from build123d import *

# Parameters (mm, degrees)
BOSS_EXTRUDE1_DEPTH     = 40
SKETCH2_R               = 1.5
CUT_EXTRUDE1_DEPTH      = 40
SKETCH3_W               = 40
SKETCH3_H               = 54.5
SKETCH3_W_2             = 29
SKETCH3_H_2             = 46.5
BOSS_EXTRUDE2_DEPTH     = 18
SKETCH4_W               = 29
SKETCH4_H               = 46.5
CUT_EXTRUDE2_DEPTH      = 40
CUT_EXTRUDE3_DEPTH      = 137.090235877
CUT_EXTRUDE3_DEPTH_BACK = 137.090235877
SKETCH5_R               = 1.55
SKETCH5_R_2             = 1.05
FILLET1_R               = 20
FILLET2_R               = 20
FILLET3_R               = 20
CHAMFER1_SIZE           = 2


# Some blends are built 0.0001 mm under size
with BuildPart() as part:
    # Sketch1 → Boss-Extrude1 (new body)
    with BuildSketch(Plane.XY):
        Polygon((-63.639610307, 63.639610307), (0, 0), (0, 6), (2.485281374, 6), (-59.39696962, 67.882250994), align=None)
        Polygon((0, 6), (0, 0), (4.242640687, 4.242640687), (2.485281374, 6), align=None)
        Polygon((4.242640687, 4.242640687), (0, 0), (65, 0), (60.757359313, 4.242640687), (62.514718626, 6), (2.485281374, 6), align=None)
        Polygon((60.757359313, 4.242640687), (65, 0), (65, 6), (62.514718626, 6), align=None)
        Polygon((65, 6), (65, 0), (110.961940777, 45.961940777), (106.71930009, 50.204581464), (62.514718626, 6), align=None)
    extrude(amount=BOSS_EXTRUDE1_DEPTH)

    # Sketch2 → Cut-Extrude1 (cut)
    with BuildSketch(Plane(origin=(28.257359313, -28.257359313, 0), x_dir=(0, 0, 1), z_dir=(-0.7071067811865464, 0.7071067811865488, 0))):
        with Locations(Location((20, 82.961940777, 0), (0, 0, 270))):
            Circle(SKETCH2_R)
        with Locations(Location((12, 90.961940777, 0), (0, 0, 270))):
            Circle(SKETCH2_R)
        with BuildLine():
            ThreePointArc((24, 90.961940777), (21.530733729, 94.657458907), (17.171572875, 93.790367902))
            Line((17.171572875, 93.790367902), (22.828427125, 88.133513652))
            ThreePointArc((22.828427125, 88.133513652), (23.69551813, 89.431207048), (24, 90.961940777))
        make_face()
        with BuildLine():
            Line((22.828427125, 88.133513652), (17.171572875, 93.790367902))
            ThreePointArc((17.171572875, 93.790367902), (17.171572875, 88.133513652), (22.828427125, 88.133513652))
        make_face()
        with Locations(Location((20, 98.961940777, 0), (0, 0, 270))):
            Circle(SKETCH2_R)
        with Locations(Location((28, 90.961940777, 0), (0, 0, 270))):
            Circle(SKETCH2_R)
    extrude(amount=-CUT_EXTRUDE1_DEPTH, mode=Mode.SUBTRACT)

    # Sketch3 → Boss-Extrude2 (add)
    with BuildSketch(Plane(origin=(0, 0, 0), x_dir=(0, 0, 1), z_dir=(-0.7071067811865464, -0.7071067811865488, 0))):
        with Locations((20, 62.75)):
            Rectangle(SKETCH3_W, SKETCH3_H)
        with Locations((20, 62.75)):
            Rectangle(SKETCH3_W_2, SKETCH3_H_2, mode=Mode.SUBTRACT)
    extrude(amount=BOSS_EXTRUDE2_DEPTH)

    # Sketch4 → Cut-Extrude2 (cut)
    with BuildSketch(Plane(origin=(0, 0, 0), x_dir=(0, 0, 1), z_dir=(-0.7071067811865464, -0.7071067811865488, 0))):
        with Locations((20, 62.75)):
            Rectangle(SKETCH4_W, SKETCH4_H)
    extrude(amount=-CUT_EXTRUDE2_DEPTH, mode=Mode.SUBTRACT)

    # Sketch5 → Cut-Extrude3 (cut, two sides: drawn at the far end of the back side and taken through both)
    # profile 1 of 8: a face of its own
    with BuildSketch(Plane.XY.offset(40).offset(-CUT_EXTRUDE3_DEPTH_BACK)):
        with Locations((-51.335952314, 48.648946546)):
            Circle(SKETCH5_R)
        with Locations((-51.335952314, 48.648946546)):
            Circle(SKETCH5_R_2, mode=Mode.SUBTRACT)
    # profile 2 of 8: a face of its own
    with BuildSketch(Plane.XY.offset(40).offset(-CUT_EXTRUDE3_DEPTH_BACK)):
        with Locations((-51.335952314, 48.648946546)):
            Circle(SKETCH5_R_2)
    # profile 3 of 8: a face of its own
    with BuildSketch(Plane.XY.offset(40).offset(-CUT_EXTRUDE3_DEPTH_BACK)):
        with Locations((-59.821233688, 40.163665171)):
            Circle(SKETCH5_R)
        with Locations((-59.821233688, 40.163665171)):
            Circle(SKETCH5_R_2, mode=Mode.SUBTRACT)
    # profile 4 of 8: a face of its own
    with BuildSketch(Plane.XY.offset(40).offset(-CUT_EXTRUDE3_DEPTH_BACK)):
        with Locations((-59.821233688, 40.163665171)):
            Circle(SKETCH5_R_2)
    # profile 5 of 8: a face of its own
    with BuildSketch(Plane.XY.offset(40).offset(-CUT_EXTRUDE3_DEPTH_BACK)):
        with Locations((-34.365389566, 31.678383797)):
            Circle(SKETCH5_R)
        with Locations((-34.365389566, 31.678383797)):
            Circle(SKETCH5_R_2, mode=Mode.SUBTRACT)
    # profile 6 of 8: a face of its own
    with BuildSketch(Plane.XY.offset(40).offset(-CUT_EXTRUDE3_DEPTH_BACK)):
        with Locations((-34.365389566, 31.678383797)):
            Circle(SKETCH5_R_2)
    # profile 7 of 8: a face of its own
    with BuildSketch(Plane.XY.offset(40).offset(-CUT_EXTRUDE3_DEPTH_BACK)):
        with Locations((-42.85067094, 23.193102423)):
            Circle(SKETCH5_R)
        with Locations((-42.85067094, 23.193102423)):
            Circle(SKETCH5_R_2, mode=Mode.SUBTRACT)
    # profile 8 of 8: a face of its own
    with BuildSketch(Plane.XY.offset(40).offset(-CUT_EXTRUDE3_DEPTH_BACK)):
        with Locations((-42.85067094, 23.193102423)):
            Circle(SKETCH5_R_2)
    extrude(amount=CUT_EXTRUDE3_DEPTH + CUT_EXTRUDE3_DEPTH_BACK, mode=Mode.SUBTRACT)

    # Fillet1
    fillet1_edges = [part.edges().sort_by_distance(p)[0] for p in [
        (0, 0, 20),
        (2.485281374, 6, 20),
        (62.514718626, 6, 20),
        (65, 0, 20),
    ]]
    fillet(fillet1_edges, radius=FILLET1_R)

    # Fillet2
    # the kernel refuses this fillet: 20 mm, written as the material it adds along each edge
    with BuildSketch(Plane(origin=(-25.102290732, 25.102290732, 0), x_dir=(0.7071067811865487, -0.7071067811865465, 0), z_dir=(0, 0, 1))) as fillet2_piece_1:
        with BuildLine():
            CenterArc((19.899748742, -20), FILLET2_R, 90, 84.260829523)
            Line((0, -18), (-0.397994975, -17.96))
            ThreePointArc((-0.397994975, -17.96), (-0.4, -9), (-0.4, 0))
            Line((-0.4, 0), (0, 0.4))
            Line((0, 0.4), (19.899748742, 0.4))
            Line((19.899748742, 0.4), (19.899748742, 0))
        make_face()
    extrude(amount=40)

    # Fillet3
    fillet3_edges = [part.edges().sort_by_distance(p)[0] for p in [
        (108.840620434, 48.083261121, 0),
        (108.840620434, 48.083261121, 40),
    ]]
    fillet(fillet3_edges, radius=FILLET3_R - 0.0001)  # a hair under: the kernel refuses the full size

    # Chamfer1
    chamfer1_edges = [part.edges().sort_by_distance(p)[0] for p in [
        (-67.882250994, 59.39696962, 0),
        (32.5, 0, 0),
        (32.5, 0, 40),
        (-8.444453914, 8.444453914, 0),
        (-31.384776311, 39.870057685, 0),
        (32.5, 6, 0),
        (80.474909089, 23.960190464, 0),
        (83.83887012, 18.83887012, 0),
        (64.3693974, 1.52240935, 0),
        (0.6306026, 1.52240935, 0),
        (-8.444453914, 8.444453914, 40),
        (83.83887012, 18.83887012, 40),
        (80.474909089, 23.960190464, 40),
        (32.5, 6, 40),
        (-31.384776311, 39.870057685, 40),
        (64.3693974, 1.52240935, 40),
        (0.6306026, 1.52240935, 40),
        (3.115883974, 7.52240935, 0),
        (3.115883974, 7.52240935, 40),
        (61.884116026, 7.52240935, 0),
        (61.884116026, 7.52240935, 40),
        (-24.171923575, 16.863829291, 40),
        (-24.171923575, 16.863829291, 0),
        (106.819825864, 41.819825864, 34.142164913),
        (106.819825864, 41.819825864, 5.857835087),
        (102.577185177, 46.062466551, 34.142164913),
        (102.577185177, 46.062466551, 5.857835087),
        (-67.882250994, 59.39696962, 40),
    ]]
    chamfer(chamfer1_edges, length=CHAMFER1_SIZE)


solid = part.part
For this review, take the finished solid that the model builds, in its own axes (mm). A direction names the side the tool comes from. Round coordinates to 2 decimals unless told otherwise and drop trailing zeros. Loops run counter-clockwise (first coordinate to the right, second up) from the corner with the lowest first, then second, coordinate; pieces in that order, holes last. Notation, with made-up numbers: (5.5, 57.25) - (53.5, 57.25) arc R30 cw to (53.5, 91.25) - close; hole circle Ø10 at (3, -31). An arc over 180 degrees is marked (long way). Use one line per item in the form item = value.
1) Wall thickness on probe 1 along X at (y, z) = (17.5, 4); probe 2 along X at (y, z) = (26, 11.5); probe 3 along X at (y, z) = (57.5, 34): over which ranges is each line inside the solid? List them lowest first.
Solutions:
probe_1 = -42.96 to -9.01, 74.01 to 82.5
probe_2 = -29.86 to -17.51, 82.51 to 91
probe_3 = -69.78 to -64.12
2) Clearance check with flat-ended pins moving along their axes: P1, Ø8, axis at x = 67.5, z = 8, coming from the -Y side; P2, Ø10, axis at y = 38.5, z = 18, coming from the -X side; P3, Ø11, axis at x = 24.5, z = 26.5, coming from the +Y side. State where each tip first meets the part, or that it passes through.
Solutions:
P1 = 1.19
P2 = 90.01
P3 = 6
3) We need section B-B on y = 54. Write out the cut boundary in (x, z).
Solutions:
outline = (-73.28, 2) - (-70.45, 0) - (-48.34, 0) - (-45.51, 2) - (-45.51, 5.5) - (-67.62, 5.5) - (-67.62, 34.5) - (-45.51, 34.5) - (-45.51, 38) - (-48.34, 40) - (-70.45, 40) - (-73.28, 38) - close
4) Mouldability with a two-part tool opening along X and no side actions: class faces 1 (the face through (104.578, 43.84, 34.297)), 2 (the face through (81.342, 23.432, 1.014)), 3 (the face through (101.11, 40.41, 21.01)), 4 (the face through (1, 2.68, 0.79)) as pulls with the +X half, pulls with the -X half, needs draft (parallel to the pull), parting line crosses it, or undercut.
Solutions:
face_1 = pulls with the +X half
face_2 = undercut
face_3 = undercut
face_4 = pulls with the -X half
5) Tool access review of faces 5 (the face through (-8, 8, 20)), 6 (the face through (62.071, 6.773, 38.764)), 7 (the face through (-48, 40, 34.5)), 8 (the face through (-32.05, 23.81, 19.8)), 9 (the face through (82.994, 26.479, 19.748)): name each direction out of +Z, -Z, +X, -X, +Y, -Y from which nothing blocks a thin tool from reaching the whole face with its end or side.
Solutions:
face_5 = +Z, -Z, -X, -Y
face_6 = +Z, +Y
face_7 = none
face_8 = -X, +Y
face_9 = +Z, -Z, +Y
6) We need section A-A on x = 47. Write out the cut boundary in (y, z).
Solutions:
outline = (0, 2) - (2, 0) - (4, 0) - (6, 2) - (6, 38) - (4, 40) - (2, 40) - (0, 38) - close
7) We need section C-C on y = 63. Write out the cut boundary in (x, z).
Solutions:
outline = (-64.28, 2) - (-61.45, 0) - (-57.34, 0) - (-54.51, 2) - (-54.51, 5.5) - (-58.62, 5.5) - (-58.62, 34.5) - (-54.51, 34.5) - (-54.51, 38) - (-57.34, 40) - (-61.45, 40) - (-64.28, 38) - close
